The model under review builds one solid part; all positions refer to its coordinate system, in mm. A direction names the side the tool comes from. Give positions to 0.01 mm unless a question says otherwise; leave off trailing zeros. Order: outer loops, then holes, each group sorted by start corner. A loop starts at its lowest first (then second) coordinate and runs counter-clockwise, first axis right, second up. Notation, with made-up numbers: (46.25, -6) - (67.25, -6) arc R25 ccw to (67.25, 32) - close; hole circle Ø9 at (2.25, 54). An arc over 180 degrees is marked (long way). Write item = value, one per line. Start each with the question number.
1. We need section A-A, the plane x = 22. Give the boundary of the cut face in (y, z).
2. We need section B-B, the plane x = 35.5. Give the boundary of the cut face in (y, z).
3. Mouldability with a two-part tool opening along Y and no side actions: class faces 1 (the flat face through (31, 295, 317)), 2 (the flat face through (23, 292.147, 312)), 3 (the flat face through (25, 305, 323)) as pulls with the +Y half, pulls with the -Y half, needs draft (parallel to the pull), parting line crosses it, or undercut.
4. Machinability: for faces 4 (the flat face through (37.235, 295.889, 329.465)), 5 (the flat face through (25.06, 294.11, 314.71)), 6 (the flat face through (18.535, 295.477, 310.555)), 7 (the flat face through (36.869, 292.282, 325.021)), which of the approach directions +Z, -Z, +X, -X, +Y, -Y give a long, thin tool a straight path to every point of the face, cutting with its end or side? Answer none if there is none.
5. We need section D-D, the plane z = 316.5. Give the boundary of the cut face in (x, y).
6. Wall thickness on probe 1 along Z at (x, y) = (24, 297.5); probe 2 along Z at (x, y) = (38, 300); probe 3 along Z at (x, y) = (26, 286.5): over which ranges is each line inside the solid? List them lowest first.
7. We need section C-C, the plane y = 302.5. Give the boundary of the cut face in (x, z), and give its area (3 significant figures).
8. For P1, Ø1.7, axis at x = 35, y = 294.5, coming from the -Z side; P2, Ø1.5, axis at x = 21.5, y = 287, coming from the -Z side; P3, Ø10, axis at x = 28.5, y = 298, coming from the -Z side, all flat-tipped, find the tip position at first contact; note any pin that passes through.
from build123d import *

# Parameters (mm, degrees)
PRISM094_DEPTH                = 30
PRISM094_PITCH_ANGLE          = 90
PRISM095_DEPTH                = 10
PRISM095_PITCH_ANGLE          = 90
PRISM096_DEPTH                = 30
PRISM096_ROLL_ANGLE           = 90
PRISM097_DEPTH                = 10
PRISM097_ROLL_ANGLE           = 90
CUBE092_W                     = 60
CUBE092_H                     = 30
CUBE092_DEPTH                 = 20
CUBE092_PLACEMENT_ANGLE       = 45
CUBE091_W                     = 30
CUBE091_H                     = 30
CUBE091_DEPTH                 = 20
DIFFERENCE055_PITCH_ANGLE     = -90
DIFFERENCE055_PLACEMENT_ANGLE = -90


with BuildPart() as prism094:
    # prism094 → prism094 (new body)
    with BuildSketch(Plane.XY):
        Polygon((1.6, 0), (1.294427, 0.940456), (0.494427, 1.52169), (-0.494427, 1.52169), (-1.294427, 0.940456), (-1.6, 0), (-1.294427, -0.940456), (-0.494427, -1.52169), (0.494427, -1.52169), (1.294427, -0.940456), align=None)
    extrude(amount=PRISM094_DEPTH)


with BuildPart() as prism094_1:
    # prism094 pitch: moved
    add(prism094.part.rotate(Axis((0, 0, 0), (0, 1, 0)), PRISM094_PITCH_ANGLE))


with BuildPart() as prism094_2:
    # prism094 placement: moved
    add(prism094_1.part.moved(Location((5, 20, 10))))


with BuildPart() as prism095:
    # prism095 → prism095 (new body)
    with BuildSketch(Plane.XY):
        Polygon((3, 0), (2.427051, 1.763356), (0.927051, 2.85317), (-0.927051, 2.85317), (-2.427051, 1.763356), (-3, 0), (-2.427051, -1.763356), (-0.927051, -2.85317), (0.927051, -2.85317), (2.427051, -1.763356), align=None)
    extrude(amount=PRISM095_DEPTH)


with BuildPart() as prism095_1:
    # prism095 pitch: moved
    add(prism095.part.rotate(Axis((0, 0, 0), (0, 1, 0)), PRISM095_PITCH_ANGLE))


with BuildPart() as prism095_2:
    # prism095 placement: moved
    add(prism095_1.part.moved(Location((15, 20, 10))))


with BuildPart() as prism096:
    # prism096 → prism096 (new body)
    with BuildSketch(Plane.XY):
        Polygon((1.6, 0), (1.294427, 0.940456), (0.494427, 1.52169), (-0.494427, 1.52169), (-1.294427, 0.940456), (-1.6, 0), (-1.294427, -0.940456), (-0.494427, -1.52169), (0.494427, -1.52169), (1.294427, -0.940456), align=None)
    extrude(amount=PRISM096_DEPTH)


with BuildPart() as prism096_1:
    # prism096 roll: moved
    add(prism096.part.rotate(Axis((0, 0, 0), (1, 0, 0)), PRISM096_ROLL_ANGLE))


with BuildPart() as prism096_2:
    # prism096 placement: moved
    add(prism096_1.part.moved(Location((10, 20, 10))))


with BuildPart() as prism097:
    # prism097 → prism097 (new body)
    with BuildSketch(Plane.XY):
        Polygon((3, 0), (2.427051, 1.763356), (0.927051, 2.85317), (-0.927051, 2.85317), (-2.427051, 1.763356), (-3, 0), (-2.427051, -1.763356), (-0.927051, -2.85317), (0.927051, -2.85317), (2.427051, -1.763356), align=None)
    extrude(amount=PRISM097_DEPTH)


with BuildPart() as prism097_1:
    # prism097 roll: moved
    add(prism097.part.rotate(Axis((0, 0, 0), (1, 0, 0)), PRISM097_ROLL_ANGLE))


with BuildPart() as prism097_2:
    # prism097 placement: moved
    add(prism097_1.part.moved(Location((10, 15, 10))))


with BuildPart() as union044:
    # cube092 → cube092 (new body)
    with BuildSketch(Plane.XY):
        with Locations((30, 15)):
            Rectangle(CUBE092_W, CUBE092_H)
    extrude(amount=CUBE092_DEPTH)


with BuildPart() as union044_1:
    # cube092 placement: moved
    add(union044.part.rotate(Axis((0, 0, 0), (0, 0, 1)), CUBE092_PLACEMENT_ANGLE))

    # union044: union prism094, prism095, prism096, prism097
    add(prism094_2.part)
    add(prism095_2.part)
    add(prism096_2.part)
    add(prism097_2.part)


with BuildPart() as difference055:
    # cube091 → cube091 (new body)
    with BuildSketch(Plane.XY):
        with Locations((15, 15)):
            Rectangle(CUBE091_W, CUBE091_H)
    extrude(amount=CUBE091_DEPTH)

    # difference055: cut union044
    add(union044_1.part, mode=Mode.SUBTRACT)


with BuildPart() as difference055_1:
    # difference055 pitch: moved
    add(difference055.part.rotate(Axis((0, 0, 0), (0, 1, 0)), DIFFERENCE055_PITCH_ANGLE))


with BuildPart() as difference055_2:
    # difference055 placement: moved
    add(difference055_1.part.moved(Location((16, 285, 302))).rotate(Axis((16, 285, 302), (0, 0, 1)), DIFFERENCE055_PLACEMENT_ANGLE))


solid = difference055_2.part
Model answer:
q1.outline = (285, 308) - (305, 308) - (305, 332) - (285, 332) - close; hole (292.15, 311.07) - (293.24, 309.57) - (295, 309) - (296.76, 309.57) - (297.85, 311.07) - (297.85, 312.93) - (296.76, 314.43) - (295, 315) - (293.24, 314.43) - (292.15, 312.93) - close
q2.outline = (285, 321.5) - (292.16, 321.5) - (292.16, 327) - (293.56, 327) - (293.56, 332) - (285, 332) - close; (296.44, 327) - (297.84, 327) - (297.84, 321.5) - (305, 321.5) - (305, 332) - (296.44, 332) - close
q3.face_1 = needs draft
q3.face_2 = undercut
q3.face_3 = pulls with the +Y half
q4.face_4 = +Z, -Z
q4.face_5 = +X
q4.face_6 = +X, -X
q4.face_7 = -Z
q5.outline = (16, 285) - (30.5, 285) - (30.5, 305) - (16, 305) - close
q6.probe_1 = 310 to 310.59, 313.41 to 332
q6.probe_2 = 324 to 332
q6.probe_3 = 312 to 332
q7.outline = (16, 302) - (46, 332) - (16, 332) - close
q7.area = 450 mm2
q8.P1 = 327
q8.P2 = 306.75
q8.P3 = 309.5
